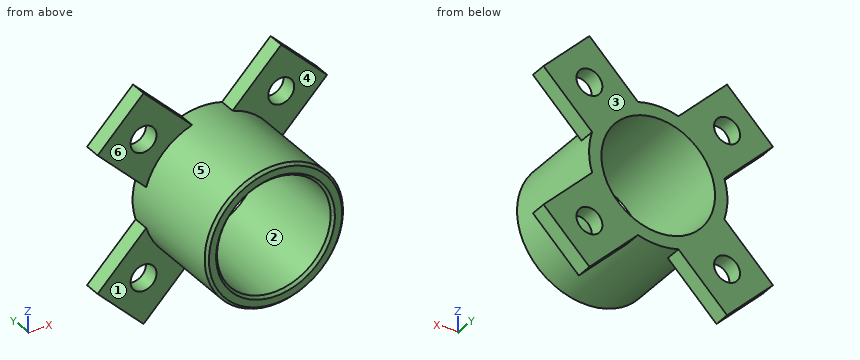
```python
from build123d import *

# Parameters (mm, degrees)
F0_R     = 1.27
F1_DEPTH = 1.5875
F2_DEPTH = 11.0500585288
F3_SIZE  = 0.254


with BuildPart() as f1:
    # F0 (on Front) → F1 (new body)
    with BuildSketch(Plane.XZ):
        with BuildLine():
            Line((-6.7335235308, -11.2269887114), (-1.9790852934, -6.4725504739))
            ThreePointArc((-1.9790852934, -6.4725504739), (-4.785952791, -4.785952791), (-6.4725504739, -1.9790852934))
            Line((-6.4725504739, -1.9790852934), (-11.2269887114, -6.7335235308))
            Line((-11.2269887114, -6.7335235308), (-6.7335235308, -11.2269887114))
        make_face()
        with Locations((-6.7335235308, -6.7368606508)):
            Circle(F0_R, mode=Mode.SUBTRACT)
        with BuildLine():
            Line((6.7351920908, -11.2253201513), (11.2253201513, -6.7351920908))
            Line((11.2253201513, -6.7351920908), (6.4717686116, -1.9816405511))
            ThreePointArc((6.4717686116, -1.9816405511), (4.785952791, -4.785952791), (1.9816405511, -6.4717686116))
            Line((1.9816405511, -6.4717686116), (6.7351920908, -11.2253201513))
        make_face()
        with Locations((6.7351920908, -6.7351920908)):
            Circle(F0_R, mode=Mode.SUBTRACT)
        with BuildLine():
            Line((-11.2253201513, 6.7351920908), (-6.4717686116, 1.9816405511))
            ThreePointArc((-6.4717686116, 1.9816405511), (-4.785952791, 4.785952791), (-1.9816405511, 6.4717686116))
            Line((-1.9816405511, 6.4717686116), (-6.7351920908, 11.2253201513))
            Line((-6.7351920908, 11.2253201513), (-11.2253201513, 6.7351920908))
        make_face()
        with Locations((-6.7351920908, 6.7351920908)):
            Circle(F0_R, mode=Mode.SUBTRACT)
        with BuildLine():
            ThreePointArc((1.9790852934, 6.4725504739), (4.785952791, 4.785952791), (6.4725504739, 1.9790852934))
            Line((6.4725504739, 1.9790852934), (11.2269887114, 6.7335235308))
            Line((11.2269887114, 6.7335235308), (6.7335235308, 11.2269887114))
            Line((6.7335235308, 11.2269887114), (1.9790852934, 6.4725504739))
        make_face()
        with Locations((6.7368606508, 6.7335235308)):
            Circle(F0_R, mode=Mode.SUBTRACT)
        with BuildLine():
            ThreePointArc((-1.9790852934, -6.4725504739), (0.0013360998, -6.7683592141), (1.9816405511, -6.4717686116))
            Line((1.9816405511, -6.4717686116), (0.9791637116, -5.4692917721))
            ThreePointArc((0.9791637116, -5.4692917721), (0.001437958, -5.5562498139), (-0.9763326742, -5.4697978547))
            Line((-0.9763326742, -5.4697978547), (-1.9790852934, -6.4725504739))
        make_face()
        with BuildLine():
            ThreePointArc((1.9816405511, -6.4717686116), (4.785952791, -4.785952791), (6.4717686116, -1.9816405511))
            Line((6.4717686116, -1.9816405511), (5.4692917721, -0.9791637116))
            ThreePointArc((5.4692917721, -0.9791637116), (3.928862053, -3.928862053), (0.9791637116, -5.4692917721))
            Line((0.9791637116, -5.4692917721), (1.9816405511, -6.4717686116))
        make_face()
        with BuildLine():
            ThreePointArc((-6.4725504739, -1.9790852934), (-4.785952791, -4.785952791), (-1.9790852934, -6.4725504739))
            Line((-1.9790852934, -6.4725504739), (-0.9763326742, -5.4697978547))
            ThreePointArc((-0.9763326742, -5.4697978547), (-3.928862053, -3.928862053), (-5.4697978547, -0.9763326742))
            Line((-5.4697978547, -0.9763326742), (-6.4725504739, -1.9790852934))
        make_face()
        with BuildLine():
            Line((5.4692917721, -0.9791637116), (6.4717686116, -1.9816405511))
            ThreePointArc((6.4717686116, -1.9816405511), (6.6938010055, -1.001856444), (6.7683593459, 0))
            ThreePointArc((6.7683593459, 0), (6.6939986454, 1.0005350428), (6.4725504739, 1.9790852934))
            Line((6.4725504739, 1.9790852934), (5.4697978547, 0.9763326742))
            ThreePointArc((5.4697978547, 0.9763326742), (5.5345947635, 0.4900763879), (5.55625, 0))
            ThreePointArc((5.55625, 0), (5.5344677464, -0.4915087251), (5.4692917721, -0.9791637116))
        make_face()
        with BuildLine():
            Line((5.4697978547, 0.9763326742), (6.4725504739, 1.9790852934))
            ThreePointArc((6.4725504739, 1.9790852934), (4.785952791, 4.785952791), (1.9790852934, 6.4725504739))
            Line((1.9790852934, 6.4725504739), (0.9763326742, 5.4697978547))
            ThreePointArc((0.9763326742, 5.4697978547), (3.928862053, 3.928862053), (5.4697978547, 0.9763326742))
        make_face()
        with BuildLine():
            Line((0.9763326742, 5.4697978547), (1.9790852934, 6.4725504739))
            ThreePointArc((1.9790852934, 6.4725504739), (-0.0013360998, 6.7683592141), (-1.9816405511, 6.4717686116))
            Line((-1.9816405511, 6.4717686116), (-0.9791637116, 5.4692917721))
            ThreePointArc((-0.9791637116, 5.4692917721), (-0.001437958, 5.5562498139), (0.9763326742, 5.4697978547))
        make_face()
        with BuildLine():
            ThreePointArc((-6.4717686116, 1.9816405511), (-6.7683592141, 0.0013360998), (-6.4725504739, -1.9790852934))
            Line((-6.4725504739, -1.9790852934), (-5.4697978547, -0.9763326742))
            ThreePointArc((-5.4697978547, -0.9763326742), (-5.5562498139, 0.001437958), (-5.4692917721, 0.9791637116))
            Line((-5.4692917721, 0.9791637116), (-6.4717686116, 1.9816405511))
        make_face()
        with BuildLine():
            ThreePointArc((-5.4692917721, 0.9791637116), (-3.928862053, 3.928862053), (-0.9791637116, 5.4692917721))
            Line((-0.9791637116, 5.4692917721), (-1.9816405511, 6.4717686116))
            ThreePointArc((-1.9816405511, 6.4717686116), (-4.785952791, 4.785952791), (-6.4717686116, 1.9816405511))
            Line((-6.4717686116, 1.9816405511), (-5.4692917721, 0.9791637116))
        make_face()
    extrude(amount=F1_DEPTH)

    # F0 (on Front) → F2 (join)
    with BuildSketch(Plane.XZ):
        with BuildLine():
            Line((5.4697978547, 0.9763326742), (6.4725504739, 1.9790852934))
            ThreePointArc((6.4725504739, 1.9790852934), (4.785952791, 4.785952791), (1.9790852934, 6.4725504739))
            Line((1.9790852934, 6.4725504739), (0.9763326742, 5.4697978547))
            ThreePointArc((0.9763326742, 5.4697978547), (3.928862053, 3.928862053), (5.4697978547, 0.9763326742))
        make_face()
        with BuildLine():
            Line((5.4692917721, -0.9791637116), (6.4717686116, -1.9816405511))
            ThreePointArc((6.4717686116, -1.9816405511), (6.6938010055, -1.001856444), (6.7683593459, 0))
            ThreePointArc((6.7683593459, 0), (6.6939986454, 1.0005350428), (6.4725504739, 1.9790852934))
            Line((6.4725504739, 1.9790852934), (5.4697978547, 0.9763326742))
            ThreePointArc((5.4697978547, 0.9763326742), (5.5345947635, 0.4900763879), (5.55625, 0))
            ThreePointArc((5.55625, 0), (5.5344677464, -0.4915087251), (5.4692917721, -0.9791637116))
        make_face()
        with BuildLine():
            ThreePointArc((1.9816405511, -6.4717686116), (4.785952791, -4.785952791), (6.4717686116, -1.9816405511))
            Line((6.4717686116, -1.9816405511), (5.4692917721, -0.9791637116))
            ThreePointArc((5.4692917721, -0.9791637116), (3.928862053, -3.928862053), (0.9791637116, -5.4692917721))
            Line((0.9791637116, -5.4692917721), (1.9816405511, -6.4717686116))
        make_face()
        with BuildLine():
            ThreePointArc((-1.9790852934, -6.4725504739), (0.0013360998, -6.7683592141), (1.9816405511, -6.4717686116))
            Line((1.9816405511, -6.4717686116), (0.9791637116, -5.4692917721))
            ThreePointArc((0.9791637116, -5.4692917721), (0.001437958, -5.5562498139), (-0.9763326742, -5.4697978547))
            Line((-0.9763326742, -5.4697978547), (-1.9790852934, -6.4725504739))
        make_face()
        with BuildLine():
            ThreePointArc((-6.4725504739, -1.9790852934), (-4.785952791, -4.785952791), (-1.9790852934, -6.4725504739))
            Line((-1.9790852934, -6.4725504739), (-0.9763326742, -5.4697978547))
            ThreePointArc((-0.9763326742, -5.4697978547), (-3.928862053, -3.928862053), (-5.4697978547, -0.9763326742))
            Line((-5.4697978547, -0.9763326742), (-6.4725504739, -1.9790852934))
        make_face()
        with BuildLine():
            ThreePointArc((-6.4717686116, 1.9816405511), (-6.7683592141, 0.0013360998), (-6.4725504739, -1.9790852934))
            Line((-6.4725504739, -1.9790852934), (-5.4697978547, -0.9763326742))
            ThreePointArc((-5.4697978547, -0.9763326742), (-5.5562498139, 0.001437958), (-5.4692917721, 0.9791637116))
            Line((-5.4692917721, 0.9791637116), (-6.4717686116, 1.9816405511))
        make_face()
        with BuildLine():
            ThreePointArc((-5.4692917721, 0.9791637116), (-3.928862053, 3.928862053), (-0.9791637116, 5.4692917721))
            Line((-0.9791637116, 5.4692917721), (-1.9816405511, 6.4717686116))
            ThreePointArc((-1.9816405511, 6.4717686116), (-4.785952791, 4.785952791), (-6.4717686116, 1.9816405511))
            Line((-6.4717686116, 1.9816405511), (-5.4692917721, 0.9791637116))
        make_face()
        with BuildLine():
            Line((0.9763326742, 5.4697978547), (1.9790852934, 6.4725504739))
            ThreePointArc((1.9790852934, 6.4725504739), (-0.0013360998, 6.7683592141), (-1.9816405511, 6.4717686116))
            Line((-1.9816405511, 6.4717686116), (-0.9791637116, 5.4692917721))
            ThreePointArc((-0.9791637116, 5.4692917721), (-0.001437958, 5.5562498139), (0.9763326742, 5.4697978547))
        make_face()
    extrude(amount=F2_DEPTH)

    # F3
    f3_edges = [f1.edges().sort_by_distance(p)[0] for p in [
        (-1.979085, -11.050059, -6.47255),
        (0.979164, -11.050059, -5.469292),
    ]]
    chamfer(f3_edges, length=F3_SIZE)


solid = f1.part
```
Build history of the part. All positions in model axes, mm. Face numbers are marked on the shaded views. A direction names the side the tool comes from. Round coordinates to 2 decimals unless told otherwise and drop trailing zeros. Loops run counter-clockwise (first coordinate to the right, second up) from the corner with the lowest first, then second, coordinate; pieces in that order, holes last.
Item 1: Saw through at A-A (z = -9.5). List the corners of the cut face in (x, y), then the cut area to 3 significant figures.
Item 2: Pin check, flat tips, straight feed: P1, Ø1.5, axis at y = -5, z = 4.5, coming from the +X side; P2, Ø3, axis at x = 7, z = 4.5, coming from the -Y side; P3, Ø1.5, axis at y = -2.5, z = -1.5, coming from the -X side. Stop position of each tip, or through.
Item 3: Saw through at C-C (y = -6.25). List the corners of the cut face in (x, z).
Item 4: Drill centre lines: line 1 along Z through (x, y) = (0, -2.25); line 2 along Z through (x, y) = (-5, -5.5); line 3 along X through (y, z) = (-5.5, 0.5). Where is each one in solid material? Low to high.
Item 5: Two-plate mould, pull along Z, no slides. Class the marked faces 1 and 2: released by +Z, released by -Z, zero draft, split by the parting line, or undercut.
Item 6: Saw through at B-B (y = -0.75). List the corners of the cut face in (x, z).
Item 7: Which spindle directions (+Z, -Z, +X, -X, +Y, -Y) get a long thin tool onto all of the face, cutting with end or side? Do the marked faces 3, 4, 5 and 6. Say none if no direction does.
Worked answers:
1. outline: (-8.46, -1.59) - (-5.01, -1.59) - (-5.01, 0) - (-8.46, 0) - close; (5.01, -1.59) - (8.46, -1.59) - (8.46, 0) - (5.01, 0) - close
1. area: 11.0 mm2
2. P1: stops at x = 5.63
2. P2: stops at y = -1.59
2. P3: stops at x = -6.73
3. outline: circle Ø13.54 at (0, 0); hole circle Ø11.11 at (0, 0)
4. line 1: z = -6.77 to -5.56, 5.56 to 6.77
4. line 2: z = -4.56 to -2.42, 2.42 to 4.56
4. line 3: x = -6.75 to -5.53, 5.53 to 6.75
5. face 1: zero draft
5. face 2: undercut
6. outline: (-11.23, -6.73) - (-6.73, -11.23) - (-1.98, -6.47) arc R6.77 ccw to (1.98, -6.47) - (6.74, -11.23) - (11.23, -6.74) - (6.47, -1.98) arc R6.77 ccw to (6.47, 1.98) - (11.23, 6.73) - (6.73, 11.23) - (1.98, 6.47) arc R6.77 ccw to (-1.98, 6.47) - (-6.74, 11.23) - (-11.23, 6.74) - (-6.47, 1.98) arc R6.77 ccw to (-6.47, -1.98) - close; hole circle Ø2.54 at (-6.74, 6.74); hole circle Ø2.54 at (-6.73, -6.74); hole circle Ø11.11 at (0, 0); hole circle Ø2.54 at (6.74, -6.74); hole circle Ø2.54 at (6.74, 6.73)
7. face 3: +Z, -Z, +X, -X, +Y
7. face 4: +Z, +X, -Y
7. face 5: -Y
7. face 6: +Z, -X, -Y
